from build123d import *

# Parameters (mm, degrees)
BOSS_EXTRUDE1_DEPTH = 14
CHAMFER1_SIZE       = 0.5
SKETCH2_W           = 3
SKETCH2_H           = 1.4
CUT_EXTRUDE1_DEPTH  = 15


with BuildPart() as part:
    # Sketch1 → Boss-Extrude1 (new body)
    with BuildSketch(Plane.XY):
        with BuildLine():
            Line((-26.871279399, 53.748878842), (-26.871279399, 52.748878842))
            Line((-26.871279399, 52.748878842), (-25.171279399, 52.748878842))
            Line((-25.171279399, 52.748878842), (-25.171279399, 53.748878842))
            ThreePointArc((-25.171279399, 53.748878842), (-23.171279399, 55.748878842), (-21.171279399, 53.748878842))
            Line((-21.171279399, 53.748878842), (-21.171279399, 52.748878842))
            Line((-21.171279399, 52.748878842), (-19.471279399, 52.748878842))
            Line((-19.471279399, 52.748878842), (-19.471279399, 53.748878842))
            Line((-19.471279399, 53.748878842), (-19.471279399, 56.548878842))
            Line((-19.471279399, 56.548878842), (-26.871279399, 56.548878842))
            Line((-26.871279399, 56.548878842), (-26.871279399, 53.748878842))
        make_face()
    extrude(amount=BOSS_EXTRUDE1_DEPTH)

    # Chamfer1
    chamfer1_edges = [part.edges().sort_by_distance(p)[0] for p in [
        (-26.871279399, 52.748878842, 7),
        (-19.471279399, 52.748878842, 7),
    ]]
    chamfer(chamfer1_edges, length=CHAMFER1_SIZE)

    # Sketch2 → Cut-Extrude1 (cut)
    with BuildSketch(Plane(origin=(-19.471279399, 0, 0), x_dir=(0, 0, -1), z_dir=(1, 0, 0))):
        with Locations((-9.5, 55.848878842)):
            Rectangle(SKETCH2_W, SKETCH2_H)
    extrude(amount=-CUT_EXTRUDE1_DEPTH, mode=Mode.SUBTRACT)


solid = part.part
Can you work these out from the model? Positions are in its coordinate system, mm. A direction names the side the tool comes from. Round coordinates to 2 decimals unless told otherwise and drop trailing zeros. Write each loop counter-clockwise with the first axis right and the second up, starting at its lowest first coordinate (ties: lowest second). Pieces come first, ordered by that corner, then holes. Notation, with made-up numbers: M 64,-29 L 102,-29 A22 ccw 102,-10 Z; hole C 42.5,27 d2. An arc over 180 degrees is marked long. Use CSV: the item, a comma, the result in double quotes.
(1) We'd pull the mould along X, two halves only. Please class faces 1 (the cylindrical face through (-23.22, 55.75, 6.9)), 2 (the flat face through (-26, 52.749, 7)), 3 (the flat face through (-19.471, 55, 7)): +X half, -X half, draft (parallel to the pull), parting line (faces both ways), or undercut.
Check values:
face 1,"undercut"
face 2,"draft"
face 3,"+X half"
(2) I'm going to push a flat-ended pin straight in: pin 1 (0.7 mm diameter, centred on x = -20.5, z = 9.5, fed in from +Y). Where does the tip first touch, or does it pass through?
Check values:
pin 1,"y = 55.15"
(3) I need wall thicknesses on line 1 along Z through (x, y) = (-20.25, 56.1); line 2 along X through (y, z) = (54.4, 6.5); line 3 along Y through (x, z) = (-20.25, 9.5). Which ranges of each line are inside material? Lowest first, please.
Check values:
line 1,"0 to 8, 11 to 14"
line 2,"-26.87 to -25.06, -21.28 to -19.47"
line 3,"52.75 to 55.15"
(4) Imagine slicing it at D-D (x = -26). Write out the boundary of the cut face in (y, z), plus the area to 3 significant figures.
Check values:
outline,"M 52.75,0 L 56.55,0 L 56.55,8 L 55.15,8 L 55.15,11 L 56.55,11 L 56.55,14 L 52.75,14 Z"
area,"49.0 mm^2"
(5) On a 3-axis mill with a long thin cutter (end or side, diameter ignored), from which of +Z, -Z, +X, -X, +Y, -Y can I reach the whole of each face in a straight line? I mean faces 4 (the flat face through (-25.171, 53, 7)), 5 (the flat face through (-23, 56, 8)), 6 (the flat face through (-23, 56, 0)). Say none if no direction works.
Check values:
face 4,"+Z, -Z, -Y"
face 5,"+X, -X, +Y"
face 6,"-Z, +X, -X, +Y, -Y"
(6) Imagine slicing it at A-A (y = 53.6). Write out the boundary of the cut face in (x, z).
Check values:
outline,"M -26.87,0 L -25.17,0 L -25.17,14 L -26.87,14 Z; M -21.17,0 L -19.47,0 L -19.47,14 L -21.17,14 Z"
(7) Imagine slicing it at B-B (z = 10.25). Write out the boundary of the cut face in (x, y), plus the area to 3 significant figures.
Check values:
outline,"M -26.87,53.25 L -26.37,52.75 L -25.17,52.75 L -25.17,53.75 A2 cw -24.6,55.15 L -26.87,55.15 Z; M -21.74,55.15 A2 cw -21.17,53.75 L -21.17,52.75 L -19.97,52.75 L -19.47,53.25 L -19.47,55.15 Z"
area,"8.41 mm^2"
(8) Imagine slicing it at C-C (x = -23). Write out the boundary of the cut face in (y, z), plus the area to 3 significant figures.
Check values:
outline,"M 55.74,0 L 56.55,0 L 56.55,8 L 55.74,8 Z; M 55.74,11 L 56.55,11 L 56.55,14 L 55.74,14 Z"
area,"8.88 mm^2"
